Autodesk Inventor part; units mm, degrees
ref_plane "YZ Plane" through (0, 0, 0) normal (1, 0, 0) x (0, 1, 0)
ref_plane "XZ Plane" through (0, 0, 0) normal (0, 1, 0) x (-1, 0, 0)
ref_plane "XY Plane" through (0, 0, 0) normal (0, 0, 1) x (1, 0, 0)
sketch "Sketch1" plane through (0, 0, 0) normal (0, 0, 1) x (1, 0, 0)
  point P0 (0, 0)
sketch "Sketch2" plane through (0, 0, 0) normal (0, 0, 1) x (1, 0, 0)
  line L0 (0, 0) -> (25, 0)
  line L1 (25, 0) -> (25, 300)
  line L2 (25, 300) -> (75, 300)
  line L3 (75, 300) -> (75, 0)
  line L4 (75, 0) -> (100, 0)
  line L5 (100, 0) -> (100, 240)
  line L6 (100, 240) -> (320, 240)
  line L7 (320, 240) -> (320, 0)
  line L8 (320, 0) -> (345, 0)
  line L9 (345, 0) -> (345, 300)
  line L10 (345, 300) -> (395, 300)
  line L11 (395, 300) -> (395, 0)
  line L12 (395, 0) -> (420, 0)
  line L13 (420, 0) -> (420, 325)
  line L14 (420, 325) -> (345, 325)
  line L15 (345, 325) -> (345, 975)
  line L16 (345, 975) -> (75, 975)
  line L17 (75, 975) -> (75, 325)
  line L18 (75, 325) -> (0, 325)
  line L19 (0, 325) -> (0, 0)
  dimension "d0" = 25
  dimension "d1" = 300
  dimension "d2" = 50
  dimension "d3" = 300
  dimension "d4" = 25
  dimension "d5" = 240
  dimension "d6" = 220
  dimension "d7" = 240
  dimension "d8" = 25
  dimension "d9" = 300
  dimension "d10" = 50
  dimension "d11" = 300
  dimension "d12" = 25
  dimension "d13" = 325
  dimension "d14" = 75
  dimension "d15" = 650
  dimension "d16" = 270
  dimension "d17" = 650
  dimension "d18" = 75
sketch "Sketch3" plane through (0, 0, 0) normal (0, 0, 1) x (1, 0, 0)
  line L0 (100, 950) -> (320, 950)
  line L1 (320, 950) -> (320, 840)
  line L2 (320, 840) -> (100, 840)
  line L3 (100, 840) -> (100, 950)
  line L4 (100, 815) -> (320, 815)
  line L5 (320, 815) -> (320, 565)
  line L6 (320, 565) -> (100, 565)
  line L7 (100, 565) -> (100, 815)
  line L8 (100, 540) -> (320, 540)
  line L9 (320, 540) -> (320, 265)
  line L10 (320, 265) -> (100, 265)
  line L11 (100, 265) -> (100, 540)
  point P0 (0, 0)
  dimension "d19" = 220
  dimension "d20" = 110
  dimension "d21" = 220
  dimension "d22" = 250
  dimension "d23" = 220
  dimension "d24" = 275
extrude "Extrusion1" add sketch "Sketch2" along normal blind 25
extrude "Extrusion2" cut sketch "Sketch3" along normal through all
sketch "Sketch4" plane through (0, 0, 25) normal (0, 0, 1) x (1, 0, 0)
  line L0 (100, 840) -> (320, 840)
  arc A0 (250, 840) -> (170, 840) centre (210, 840) ccw
  point P0 (0, 0)
extrude "Extrusion3" add sketch "Sketch4" against normal blind 25
sketch "Sketch5" plane through (0, 0, 25) normal (0, 0, 1) x (1, 0, 0)
  point P0 (0, 0)
sketch "Sketch6" plane through (0, 0, 25) normal (0, 0, 1) x (1, 0, 0)
  line L0 (320, 265) -> (100, 265)
  arc A0 (250, 265) -> (170, 265) centre (210, 265) ccw
  point P0 (0, 0)
  dimension "d31" = 40
extrude "Extrusion4" add sketch "Sketch6" against normal blind 25
sketch "Sketch7" plane through (0, 0, 25) normal (0, 0, 1) x (1, 0, 0)
  line L0 (170, 265) -> (100, 265)
  line L1 (152, 265) -> (270, 265)
  line L2 (270, 265) -> (270, 251)
  line L3 (270, 251) -> (152, 251)
  line L4 (152, 251) -> (152, 265)
  point P0 (0, 0)
extrude "Extrusion5" add sketch "Sketch7" along normal blind 70
sketch "Sketch8" plane through (100, 265, 25) normal (0, 1, 0) x (1, 0, 0)
  point P0 (-100, 25)
sketch "Sketch9" plane through (100, 265, 25) normal (0, 1, 0) x (1, 0, 0)
  line L0 (64, -7) -> (71, -7)
  line L1 (71, -7) -> (71, -28)
  line L2 (71, -28) -> (64, -28)
  line L3 (64, -28) -> (64, -7)
  line L4 (64, -38) -> (71, -38)
  line L5 (71, -38) -> (71, -60)
  line L6 (71, -60) -> (64, -60)
  line L7 (64, -60) -> (64, -38)
  line L8 (149, -7) -> (156, -7)
  line L9 (156, -7) -> (156, -28)
  line L10 (156, -28) -> (149, -28)
  line L11 (149, -28) -> (149, -7)
  line L12 (148, -35) -> (156, -35)
  line L13 (156, -35) -> (156, -60)
  line L14 (156, -60) -> (148, -60)
  line L15 (148, -60) -> (148, -35)
  point P0 (-100, 25)
extrude "Extrusion6" cut sketch "Sketch9" against normal through all
sketch "Sketch10" plane through (0, 0, 25) normal (0, 0, 1) x (1, 0, 0)
  circle A0 centre (210, 280) radius 6
  point P0 (0, 0)
  dimension "d38" = 12
sketch "Sketch11" plane through (0, 0, 25) normal (0, 0, 1) x (1, 0, 0)
  circle A0 centre (210, 855) radius 6
  point P0 (0, 0)
  dimension "d39" = 12
extrude "Extrusion7" cut sketch "Sketch11" against normal through all
extrude "Extrusion8" cut sketch "Sketch10" against normal through all
properties part number "Frame_final"
For this review, take the finished solid that the model builds, in its own axes (mm). A direction names the side the tool comes from. Give positions to 0.01 mm unless a question says otherwise; leave off trailing zeros. Write each loop counter-clockwise with the first axis right and the second up, starting at its lowest first coordinate (ties: lowest second). Pieces come first, ordered by that corner, then holes. Notation, with made-up numbers: M -30,28 L 26,28 A14 ccw 26,33 Z; hole C 12.5,71 d5. An arc over 180 degrees is marked long. Answer as a JSON object with one key per item and string values. Group by question number.
Item 1: For pin 1 Ø20 at (x, z) = (240.5, 16.5) entering from -Y; pin 2 Ø7.5 at (x, z) = (398.5, 17) entering from +Y; pin 3 Ø7 at (y, z) = (259.5, 71.5) entering from +X; pin 4 Ø12 at (x, z) = (298, 35.5) entering from -Y, all flat-tipped, find the tip position at first contact; note any pin that passes through.
Item 2: Consider section B-B on y = 528.5. Write out the cut boundary in (x, z).
Item 3: Tool access review of faces 1 (the flat face through (75, 655, 12)), 2 (the flat face through (395, 152, 12)), 3 (the flat face through (320, 404, 12)): name each direction out of +Z, -Z, +X, -X, +Y, -Y from which nothing blocks a thin tool from reaching the whole face with its end or side.
Item 4: Draft analysis for pull direction X (two halves, no side actions). For faces 4 (the flat face through (420, 160, 12)), 5 (the flat face through (212, 251, 60)), 6 (the cylindrical face through (210.88, 304.99, 12.68)), state which applies: +X half, -X half, draft (parallel to the pull), parting line (faces both ways), or undercut.
Item 5: For probe 1 along Y at (x, z) = (210, 12); probe 2 along Y at (x, z) = (269.5, 18); probe 3 along X at (y, z) = (855, 9), list the stretches that pass through material, from the lowest coordinate up. Write a range as [from, to].
Item 6: Consider section C-C on z = 42.5. Write out the cut boundary in (x, y), plus the area to 3 significant figures.
Item 7: Consider section D-D on x = 285. Write out the cut boundary in (y, z).
Item 8: Consider section A-A on y = 96. Write out the cut boundary in (x, z), plus the area to 3 significant figures.
Check result:
{
 "1": {"pin 1": "stops at y = 240", "pin 2": "stops at y = 325", "pin 3": "stops at x = 270", "pin 4": "passes through"},
 "2": {"outline": "M 75,0 L 100,0 L 100,25 L 75,25 Z; M 320,0 L 345,0 L 345,25 L 320,25 Z"},
 "3": {"face 1": "+Z, -Z, -X, +Y", "face 2": "+Z, -Z, -Y", "face 3": "+Z, -Z"},
 "4": {"face 4": "+X half", "face 5": "draft", "face 6": "undercut"},
 "5": {"probe 1": "y = [240, 274], [286, 305], [540, 565], [815, 849], [861, 880], [950, 975]", "probe 2": "y = [240, 265], [540, 565], [815, 840], [950, 975]", "probe 3": "x = [75, 100], [172.92, 204], [216, 247.08], [320, 345]"},
 "6": {"outline": "M 152,251 L 164,251 L 164,265 L 152,265 Z; M 171,251 L 249,251 L 249,265 L 171,265 Z; M 256,251 L 270,251 L 270,265 L 256,265 Z", "area": "1,460 mm^2"},
 "7": {"outline": "M 240,0 L 265,0 L 265,25 L 240,25 Z; M 540,0 L 565,0 L 565,25 L 540,25 Z; M 815,0 L 840,0 L 840,25 L 815,25 Z; M 950,0 L 975,0 L 975,25 L 950,25 Z"},
 "8": {"outline": "M 0,0 L 25,0 L 25,25 L 0,25 Z; M 75,0 L 100,0 L 100,25 L 75,25 Z; M 320,0 L 345,0 L 345,25 L 320,25 Z; M 395,0 L 420,0 L 420,25 L 395,25 Z", "area": "2,500 mm^2"}
}
